Input: part model. Units: mm. Frame: model coordinates. A direction names the side the tool comes from. Round coordinates to 2 decimals unless told otherwise and drop trailing zeros. Return JSON: item names as keys, results as strings. Group by question number.
1) Mould query, pull axis Y, two halves, no side actions, for faces 1 (the face through (4, -250, 25)), 2 (the face through (257, -210.178, 33)), 3 (the face through (4, 250, 25)), 4 (the face through (4, -3, 0)). Classes: +Y half, -Y half, draft (parallel to the pull), parting line (faces both ways), or undercut.
2) Contact query for a flat-ended pin moving along its axis: P1, Ø7.5, axis at y = -195, z = 27.5, coming from the +X side. Output: stop coordinate, or through.
3) Access query for faces 5 (the face through (4, 3, 50)), 6 (the face through (257, -185.178, 34)). Directions: +Z, -Z, +X, -X, +Y, -Y. A direction counts if a zero-diameter tool reaches every point of the face in a straight line with its end or side. Return the directions, or none.
from build123d import *

# Parameters (mm, degrees)
F0_W     = 500
F0_H     = 500
F1_DEPTH = 50
F3_DEPTH = 15


with BuildPart() as f1:
    # F0 (on Top) → F1 (new body)
    with BuildSketch(Plane.XY):
        Rectangle(F0_W, F0_H)
    extrude(amount=F1_DEPTH)

    # F2 (on face) → F3 (join)
    with BuildSketch(Plane.YZ.offset(250)):
        with BuildLine():
            Line((-185.177746, 42.257256), (-185.177746, 17.257256))
            ThreePointArc((-185.177746, 17.257256), (-197.677746, 4.757256), (-210.177746, 17.257256))
            Line((-210.177746, 17.257256), (-210.177746, 42.257256))
            Line((-210.177746, 42.257256), (-210.177746, 50))
            Line((-210.177746, 50), (-250, 50))
            Line((-250, 50), (-250, 0))
            Line((-250, 0), (250, 0))
            Line((250, 0), (250, 50))
            Line((250, 50), (-185.177746, 50))
            Line((-185.177746, 50), (-185.177746, 42.257256))
        make_face()
    extrude(amount=F3_DEPTH)


solid = f1.part
Returned:
{
 "1": {"face 1": "-Y half", "face 2": "undercut", "face 3": "+Y half", "face 4": "draft"},
 "2": {"P1": "stops at x = 250"},
 "3": {"face 5": "+Z, +X, -X, +Y, -Y", "face 6": "+Z, +X"}
}
